Part print with two shaded views. Sizes in mm from the minimum x, y, z corner. A direction names the side the tool comes from. Coordinates: 2 decimals unless noted, no trailing zeros. Loops run counter-clockwise (first coordinate to the right, second up) from the corner with the lowest first, then second, coordinate; pieces in that order, holes last.
Item 1: Cut at B-B (y = 6.5). List the corners of the cut face in (x, z), and give its area (3 significant figures).
Item 2: Drill centre lines: line 1 along X through (y, z) = (4.75, 20.5); line 2 along X through (y, z) = (2.05, 20.5); line 3 along Y through (x, z) = (31, 7.5). Where is each one in solid material? Low to high.
Item 3: 3-axis set-ups, long thin cutter, end or side, ignore diameter. For the marked faces 4 and 5: which of +Z, -Z, +X, -X, +Y, -Y reach the whole face in a straight line?
Item 4: Cut at A-A (x = 20.5). List the corners of the cut face in (y, z).
Item 5: Cut at D-D (y = 1). List the corners of the cut face in (x, z) (1 decimal).
Item 6: Cut at C-C (z = 26.5). List the corners of the cut face in (x, y) (1 decimal).
Item 7: Mould opens along X. For the marked faces 1, 2 and 3 say: released by +X, released by -X, zero draft, split by the parting line, or undercut.
Item 8: Flat gauge pins, fed straight in: pin 1 (4 mm diameter, centred on x = 13, z = 10, fed in from +Y); pin 2 (2 mm diameter, centred on x = 6.53, z = 21.49, fed in from +Y); pin 3 (1.5 mm diameter, centred on x = 29, y = 4.5, fed in from -Z) (1 decimal); pin 4 (1.5 mm diameter, centred on x = 24.5, y = 1.5, fed in from -Z). Where does each tip first touch, or does it go through?
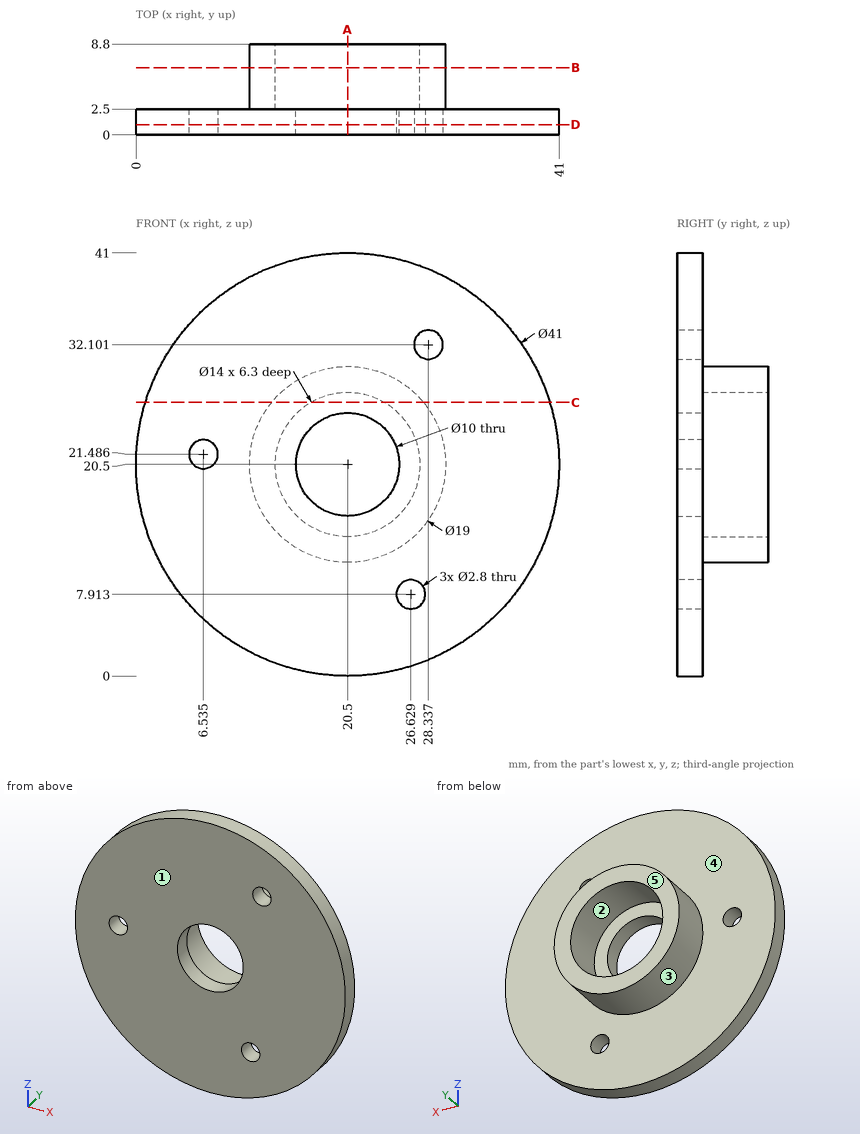
Filled sheet:
1. outline: circle Ø19 at (20.5, 20.5); hole circle Ø14 at (20.5, 20.5)
1. area: 130 mm2
2. line 1: x = 11 to 13.5, 27.5 to 30
2. line 2: x = 0 to 5.54, 7.53 to 15.5, 25.5 to 41
2. line 3: y = 0 to 2.5
3. face 4: +Y
3. face 5: +Z, -Z, +X, -X, +Y
4. outline: (0, 0) - (2.5, 0) - (2.5, 11) - (8.8, 11) - (8.8, 13.5) - (2.5, 13.5) - (2.5, 15.5) - (0, 15.5) - close; (0, 25.5) - (2.5, 25.5) - (2.5, 27.5) - (8.8, 27.5) - (8.8, 30) - (2.5, 30) - (2.5, 41) - (0, 41) - close
5. outline: circle Ø41 at (20.5, 20.5); hole circle Ø2.8 at (6.5, 21.5); hole circle Ø10 at (20.5, 20.5); hole circle Ø2.8 at (26.6, 7.9); hole circle Ø2.8 at (28.3, 32.1)
6. outline: (0.9, 0) - (40.1, 0) - (40.1, 2.5) - (27.9, 2.5) - (27.9, 8.8) - (24.1, 8.8) - (24.1, 2.5) - (16.9, 2.5) - (16.9, 8.8) - (13.1, 8.8) - (13.1, 2.5) - (0.9, 2.5) - close
7. face 1: zero draft
7. face 2: undercut
7. face 3: split by the parting line
8. pin 1: stops at y = 2.5
8. pin 2: passes through
8. pin 3: stops at z = 15
8. pin 4: stops at z = 0.26
